The figure shows three views and two pictorial views of one solid part (mm, origin at its lowest corner). Answer the questions. Give positions to 0.01 mm unless a question says otherwise; leave off trailing zeros. Loops run counter-clockwise (first coordinate to the right, second up) from the corner with the lowest first, then second, coordinate; pieces in that order, holes last. Notation, with made-up numbers: M -9,45 L 49,45 A11 cw 49,58 Z; hole C -22.75,80 d11. An arc over 180 degrees is marked long. One line per item, written item: value. Start each with the question number.
Q1. A cutting plane is placed at C-C, the plane z = 7.5. Determine the outline of the cut face in (x, y) (1 decimal), and give its area (3 significant figures).
Q2. The mould has two halves that part along X. Classify the marked faces 1, 2 and 3: +X half, -X half, draft (parallel to the pull), parting line (faces both ways), or undercut.
Q3. A cutting plane is placed at B-B, the plane y = 13. Determine the outline of the cut face in (x, z) (1 decimal), and give its area (3 significant figures).
Q4. A cutting plane is placed at A-A, the plane x = 18. Determine the outline of the cut face in (y, z).
Q5. A cutting plane is placed at D-D, the plane x = 10.75. Determine the outline of the cut face in (y, z), and give its area (3 significant figures).
Q6. Flat-ended cylindrical pins translate along their axes: pin 1 (3 mm diameter, centred on x = 13, z = 7.5, fed in from -Y); pin 2 (1 mm diameter, centred on x = 6.5, y = 4.5, fed in from +Z); pin 3 (1.5 mm diameter, centred on x = 19, z = 3, fed in from +Y); pin 4 (6 mm diameter, centred on y = 14.5, z = 4.5, fed in from +X) (1 decimal). Find the tip coordinate at first contact, or state that the pin passes through.
Q7. Consider L1, parallel to X at y = 12, z = 5.25 (1 decimal); L2, parallel to X at y = 13.25, z = 1.5 (1 decimal); L3, parallel to Y at x = 20.75, z = 6.25. Determine where each line is inside the solid, lowest interval first.
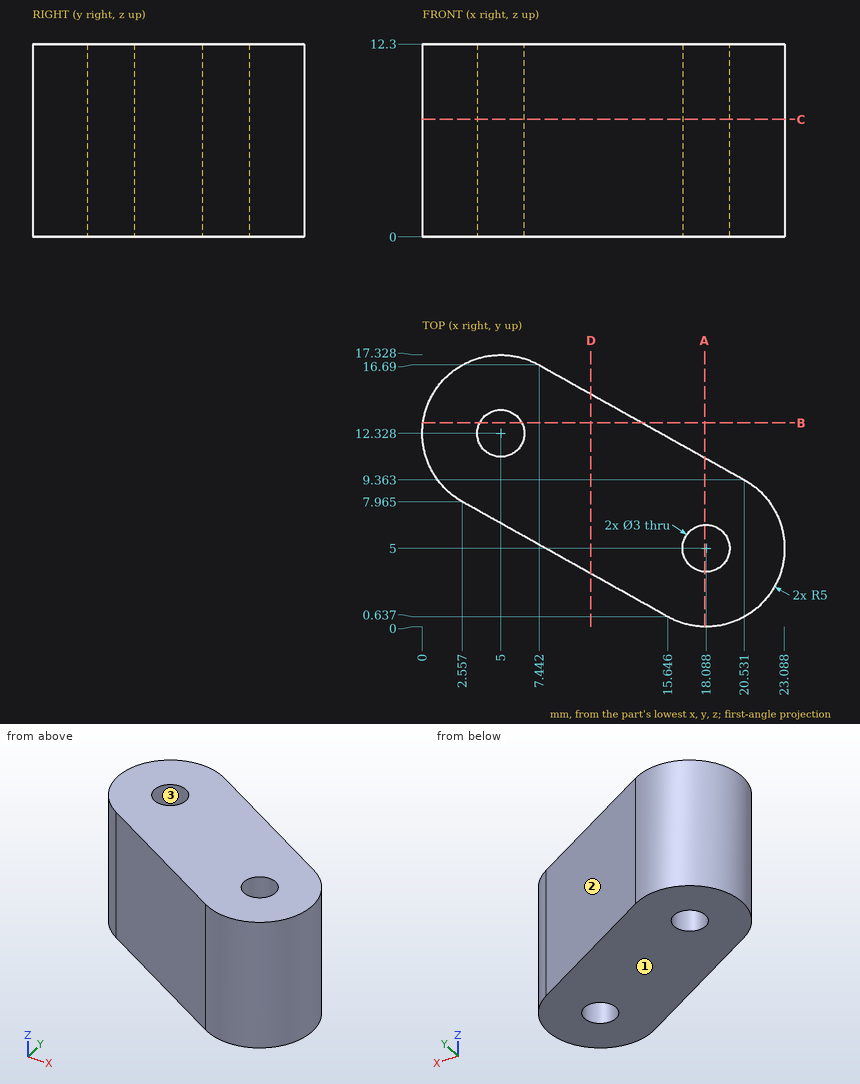
Answer block:
1. outline: M 2.6,8 L 15.6,0.6 A5 ccw 20.5,9.4 L 7.4,16.7 A5 ccw Z; hole C 5,12.3 d3; hole C 18.1,5 d3
1. area: 214 mm^2
2. face 1: draft
2. face 2: +X half
2. face 3: undercut
3. outline: M 0,0 L 3.7,0 L 3.7,12.3 L 0,12.3 Z; M 6.3,0 L 14,0 L 14,12.3 L 6.3,12.3 Z
3. area: 139 mm^2
4. outline: M 0,0 L 3.5,0 L 3.5,12.3 L 0,12.3 Z; M 6.5,0 L 10.78,0 L 10.78,12.3 L 6.5,12.3 Z
5. outline: M 3.38,0 L 14.84,0 L 14.84,12.3 L 3.38,12.3 Z
5. area: 141 mm^2
6. pin 1: y = 1.28
6. pin 2: through
6. pin 3: y = 10.64
6. pin 4: x = 16.7
7. L1: 0 to 3.5, 6.5 to 15.8
7. L2: 0.1 to 3.8, 6.2 to 13.6
7. L3: 0.77 to 9.23
